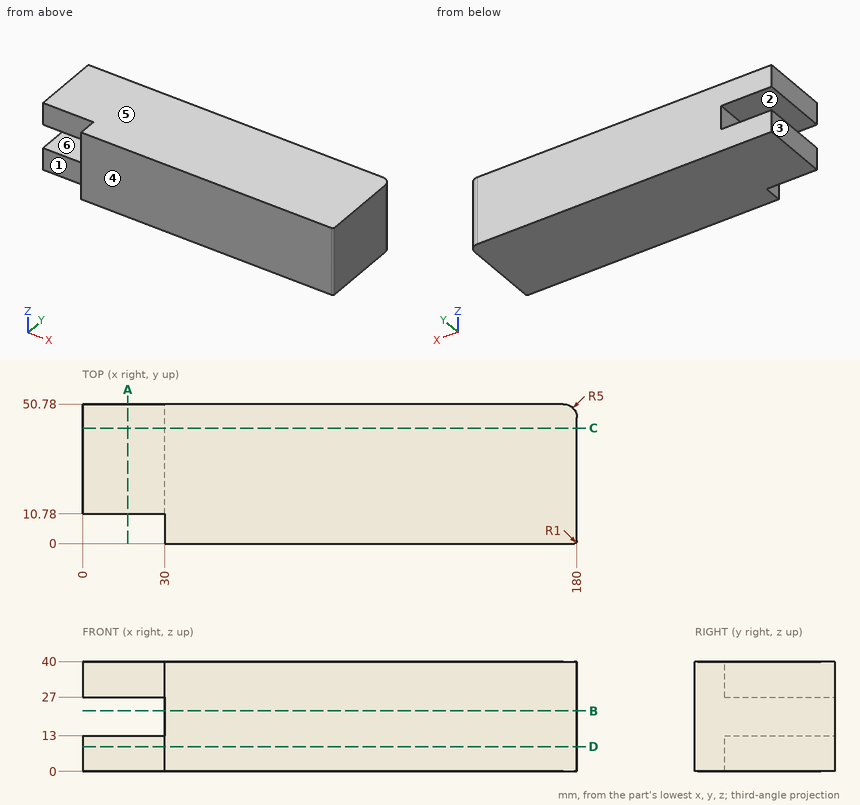
Verification items for this drawing (mm, ordinates from the low corner). A direction names the side the tool comes from. Coordinates: 2 decimals unless noted, no trailing zeros. Write each loop counter-clockwise with the first axis right and the second up, starting at its lowest first coordinate (ties: lowest second). Pieces come first, ordered by that corner, then holes. Notation, with made-up numbers: M -9.5,15 L 29.5,15 A25 ccw 29.5,27 Z; hole C -35,83.25 d5. An arc over 180 degrees is marked long. Answer as a JSON object with one key per item and string values.
1. Section check D-D, the plane z = 9. Enter the section's corners in (x, y).
Answers below:
{"outline": "M 0,10.78 L 30,10.78 L 30,0 L 179,0 A1 ccw 180,1 L 180,45.78 A5 ccw 175,50.78 L 0,50.78 Z"}
2. Draft check along Z on the marked faces 4, 5 and 6. Enter one of: released by +Z, released by -Z, zero draft, split by the parting line, or undercut.
Answers below:
{"face 4": "zero draft", "face 5": "released by +Z", "face 6": "undercut"}
3. Tool access check on the marked faces 1, 2 and 3. Record the directions out of +Z, -Z, +X, -X, +Y, -Y that give a thin tool (end or side, any length) a straight path to the whole face; none if there is none.
Answers below:
{"face 1": "+Z, -Z, -X, -Y", "face 2": "-X, +Y, -Y", "face 3": "+Z, -Z, -X, +Y, -Y"}
4. Section check B-B, the plane z = 22. Enter the section's corners in (x, y).
Answers below:
{"outline": "M 30,0 L 179,0 A1 ccw 180,1 L 180,45.78 A5 ccw 175,50.78 L 30,50.78 Z"}
5. Section check C-C, the plane y = 42. Enter the section's corners in (x, z), plus the area to 3 significant figures.
Answers below:
{"outline": "M 0,0 L 180,0 L 180,40 L 0,40 L 0,27 L 30,27 L 30,13 L 0,13 Z", "area": "6,780 mm²"}
6. Scan lines: L1, parallel to X at y = 25.5, z = 22; L2, parallel to Z at x = 8.5, y = 11; L3, parallel to Y at x = 26, z = 10.5. Record each from-to range of solid material in increasing order.
Answers below:
{"L1": "x = 30 to 180", "L2": "z = 0 to 13, 27 to 40", "L3": "y = 10.78 to 50.78"}
7. Go/stop test with flat-tipped pins: pin 1 Ø10.5 at (x, z) = (18.5, 9.5) entering from -Y; pin 2 Ø1 at (y, z) = (43, 19.5) entering from -X. Record where each tip stops, or that it passes through.
Answers below:
{"pin 1": "stops at y = 10.78", "pin 2": "stops at x = 30"}
8. Section check A-A, the plane x = 16.5. Enter the section's corners in (y, z).
Answers below:
{"outline": "M 10.78,0 L 50.78,0 L 50.78,13 L 10.78,13 Z; M 10.78,27 L 50.78,27 L 50.78,40 L 10.78,40 Z"}
